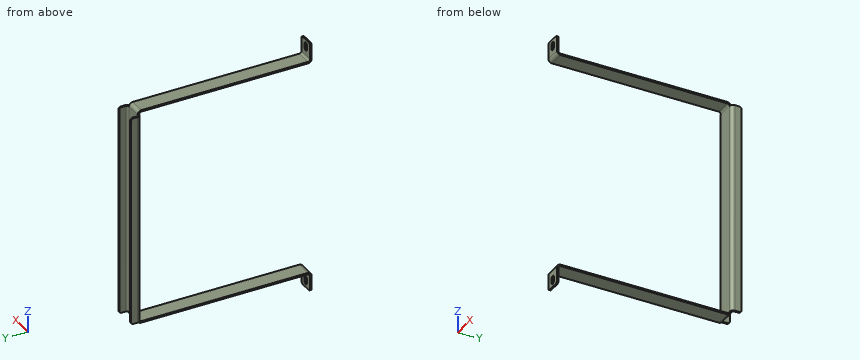
```python
from build123d import *

# Parameters (mm, degrees)
ODGI_CIE_BAZOWE1_DEPTH        = 10
ODGI_CIE_KRAW_DZI1_DEPTH      = 269.8
ODGI_CIE_KRAW_DZI1_BEND_DEPTH = 269.8
SZCZELINA_START               = -220
SZCZELINA_POD_RUB_M51_DEPTH   = 2
ZAOKR_GLENIE1_R               = 3


# Read off the part's stored shape, not the designer's step: Szczelina pod śrubę M51
# Sheet-metal steps are written as plain solids
with BuildPart() as part:
    # Szkic1 → Odgięcie bazowe1 (new, symmetric)
    with BuildSketch(Plane(origin=(0, 0, 0), x_dir=(0, 0, -1), z_dir=(1, 0, 0))):
        with BuildLine():
            Line((-162.5, -220), (-142.1, -220))
            ThreePointArc((-142.1, -220), (-138.847308807, -218.652691193), (-137.5, -215.4))
            Line((-137.5, -215.4), (-137.5, -2.6))
            ThreePointArc((-137.5, -2.6), (-136.738477631, -0.761522369), (-134.9, 0))
            Line((-134.9, 0), (134.9, 0))
            ThreePointArc((134.9, 0), (136.738477631, -0.761522369), (137.5, -2.6))
            Line((137.5, -2.6), (137.5, -215.4))
            ThreePointArc((137.5, -215.4), (138.847308807, -218.652691193), (142.1, -220))
            Line((142.1, -220), (162.5, -220))
            Line((162.5, -220), (162.5, -218))
            Line((162.5, -218), (142.1, -218))
            ThreePointArc((142.1, -218), (140.261522369, -217.238477631), (139.5, -215.4))
            Line((139.5, -215.4), (139.5, -2.6))
            ThreePointArc((139.5, -2.6), (138.152691193, 0.652691193), (134.9, 2))
            Line((134.9, 2), (-134.9, 2))
            ThreePointArc((-134.9, 2), (-138.152691193, 0.652691193), (-139.5, -2.6))
            Line((-139.5, -2.6), (-139.5, -215.4))
            ThreePointArc((-139.5, -215.4), (-140.261522369, -217.238477631), (-142.1, -218))
            Line((-142.1, -218), (-162.5, -218))
            Line((-162.5, -218), (-162.5, -220))
        make_face()
    extrude(amount=ODGI_CIE_BAZOWE1_DEPTH, both=True)

    # Odgięcie krawędzi1 section (across the edge) → Odgięcie krawędzi1 (add)
    with BuildSketch(Plane(origin=(12.6, 2, 134.9), x_dir=(-1, 0, 0), z_dir=(0, 0, -1))):
        with BuildLine():
            Line((-2, 2.6), (-2, 11))
            Line((-2, 11), (0, 11))
            Line((0, 11), (0, 2.6))
            ThreePointArc((0, 2.6), (0.761522369, 0.761522369), (2.6, 0))
            Line((2.6, 0), (2.6, -2))
            ThreePointArc((2.6, -2), (-0.652691193, -0.652691193), (-2, 2.6))
        make_face()
    extrude(amount=ODGI_CIE_KRAW_DZI1_DEPTH)

    # Odgięcie krawędzi1 section 2 (across the edge) → Odgięcie krawędzi1 bend (add)
    with BuildSketch(Plane(origin=(-12.6, 2, -134.9), x_dir=(1, 0, 0), z_dir=(0, 0, 1))):
        with BuildLine():
            Line((-2, 2.6), (-2, 11))
            Line((-2, 11), (0, 11))
            Line((0, 11), (0, 2.6))
            ThreePointArc((0, 2.6), (0.761522369, 0.761522369), (2.6, 0))
            Line((2.6, 0), (2.6, -2))
            ThreePointArc((2.6, -2), (-0.652691193, -0.652691193), (-2, 2.6))
        make_face()
    extrude(amount=ODGI_CIE_KRAW_DZI1_BEND_DEPTH)

    # Szczelina pod śrubę M51 outline → Szczelina pod śrubę M51 (cut)
    with BuildSketch(Plane(origin=(0, 0, 0), x_dir=(1, 0, 0), z_dir=(0, 1, 0)).offset(SZCZELINA_START)):
        with BuildLine():
            Line((2.75, 151), (2.75, 156))
            ThreePointArc((2.75, 156), (0, 158.75), (-2.75, 156))
            Line((-2.75, 156), (-2.75, 151))
            ThreePointArc((-2.75, 151), (0, 148.25), (2.75, 151))
        make_face()
        with BuildLine():
            ThreePointArc((2.75, -151), (0, -148.25), (-2.75, -151))
            Line((-2.75, -151), (-2.75, -156))
            ThreePointArc((-2.75, -156), (0, -158.75), (2.75, -156))
            Line((2.75, -156), (2.75, -151))
        make_face()
    extrude(amount=SZCZELINA_POD_RUB_M51_DEPTH, mode=Mode.SUBTRACT)

    # Zaokrąglenie1
    zaokr_glenie1_edges = [part.edges().sort_by_distance(p)[0] for p in [
        (-13.6, 13, 134.9),
        (-10, -219, -162.5),
        (-10, -219, 162.5),
        (10, -219, -162.5),
        (13.6, 13, 134.9),
        (13.6, 13, -134.9),
        (10, -219, 162.5),
        (-13.6, 13, -134.9),
    ]]
    fillet(zaokr_glenie1_edges, radius=ZAOKR_GLENIE1_R)


solid = part.part
```
Input: part model. Units: mm. Frame: model coordinates. Give positions to 0.01 mm unless a question says otherwise; leave off trailing zeros. Write each loop counter-clockwise with the first axis right and the second up, starting at its lowest first coordinate (ties: lowest second). Pieces come first, ordered by that corner, then holes. Notation, with made-up numbers: (60, 52) - (74, 52) arc R21 cw to (74, 77) - close; hole circle Ø10 at (26.5, 49.5). An arc over 180 degrees is marked (long way). Write item = value, one per line. Start each with the question number.
1. First-contact query: pin 1 Ø1 at (y, z) = (-219, -154) entering from -X; pin 2 Ø12 at (x, y) = (-7, -49) entering from -Z; pin 3 Ø8 at (x, y) = (3, -191.5) entering from +Z; pin 4 Ø1.4 at (x, y) = (11.5, 6) entering from -Z. Flat tips, straight axial feed; report the tip coordinate or a pass-through.
2. Ray query, L1, parallel to Z at x = 2, y = -4.5; L2, parallel to Y at x = -1.25, z = 125; L3, parallel to X at y = 2.5, z = -115. Return the intervals inside material, ascending.
3. Section query A-A, the plane y = -26. Output: boundary loops of the cut face in (x, z).
4. Section query B-B, the plane z = 113.5. Output: boundary loops of the cut face in (x, y).
Check sheet entries:
q1.pin_1 = -10
q1.pin_2 = -139.5
q1.pin_3 = 139.5
q1.pin_4 = through
q2.L1 = -139.5 to -137.5, 137.5 to 139.5
q2.L2 = 0 to 2
q2.L3 = -14.09 to -11.53, 11.53 to 14.09
q3.outline = (-10, -139.5) - (10, -139.5) - (10, -137.5) - (-10, -137.5) - close; (-10, 137.5) - (10, 137.5) - (10, 139.5) - (-10, 139.5) - close
q4.outline = (-14.6, 4.6) arc R4.6 ccw to (-10, 0) - (10, 0) arc R4.6 ccw to (14.6, 4.6) - (14.6, 13) - (12.6, 13) - (12.6, 4.6) arc R2.6 cw to (10, 2) - (-10, 2) arc R2.6 cw to (-12.6, 4.6) - (-12.6, 13) - (-14.6, 13) - close
